Build history of the part. All positions in model axes, mm. A direction names the side the tool comes from. Coordinates: 2 decimals unless noted, no trailing zeros. Loops run counter-clockwise (first coordinate to the right, second up) from the corner with the lowest first, then second, coordinate; pieces in that order, holes last.
(1) Tool access for faces 1 (the face through (3.113, 21, 75)), 2 (the face through (2.98, -5.72, 35.74)), 3 (the face through (21, -3.014, 75)), 4 (the face through (-11.93, -17.92, 75.04)), 5 (the face through (-16.65, 13.33, 75.04)): list every direction of +Z, -Z, +X, -X, +Y, -Y with a clear straight run to the whole face (end or side of a thin tool).
(2) Slice it at B-B (y = 21). Give the cut face in (x, z).
(3) Slice it at C-C (y = 5). Give the cut face in (x, z), and give its area (3 significant figures).
(4) Slice it at D-D (z = 24). Give the cut face in (x, y).
(5) Wall check: L1, parallel to Z at x = 0, y = -29; L2, parallel to X at y = 0.5, z = 34.5; L3, parallel to Y at x = 3.5, z = 53. Give the ranges that are in metal, low to high.
(6) Two-plate mould, pull along Y, no slides. Class faces 6 (the face through (-22, -3.014, 75)), 7 (the face through (-3.113, -21, 75)), 8 (the face through (12.71, 18.56, 75.04)): pulls with the +Y half, pulls with the -Y half, needs draft (parallel to the pull), parting line crosses it, or undercut.
(7) Slice it at A-A (x = 11). Give the cut face in (y, z), and give its area (3 significant figures).
(8) Flat gauge pins, fed straight in: P1, Ø1.5, axis at x = -16.5, z = 74, coming from the -Y side; P2, Ø6, axis at x = 3.5, z = -1.5, coming from the -Y side; P3, Ø1.5, axis at x = 18.5, z = 76, coming from the -Y side; P4, Ø8, axis at x = 11.5, z = 65, coming from the +Y side. Where does each tip first touch, or does it go through?
from build123d import *

# Parameters (mm, degrees)
F0_R     = 6.448973
F1_DEPTH = 75
F3_DEPTH = 2.5
F4_R     = 0.829457
F5_DEPTH = 10
F6_R     = 2.985261
F7_DEPTH = 2


with BuildPart() as f1:
    # F0 (on Top) → F1 (new body)
    with BuildSketch(Plane.XY):
        Circle(F0_R)
    extrude(amount=F1_DEPTH)

    # F2 (on face) → F3 (join, symmetric)
    with BuildSketch(Plane.XY.offset(75)):
        Polygon((7.441463, -3.014468), (35.017251, -3.014468), (35.017251, 3.014468), (8.35262, 3.014468), (27.479934, 22.758793), (22.040198, 28.188686), (3.112997, 8.650931), (3.112997, 33.119855), (-3.112997, 33.119855), (-3.112997, 9.167791), (-19.670232, 28.278624), (-25.342984, 23.363868), (-7.712681, 3.014468), (-35.017251, 3.014468), (-35.017251, -3.014468), (-8.187858, -3.014468), (-26.021978, -21.423882), (-20.502207, -26.77116), (-3.112997, -8.821007), (-3.112997, -33.119855), (3.112997, -33.119855), (3.112997, -9.480839), (20.888046, -29.997309), (26.634359, -25.167458), align=None)
    extrude(amount=F3_DEPTH, both=True)

    # F4 (on face) → F5 (join)
    with BuildSketch(Plane(origin=(0, 0, 0), x_dir=(1, 0, 0), z_dir=(0, 0, -1))):
        Circle(F4_R)
    extrude(amount=F5_DEPTH)

    # F6 (on face) → F7 (join)
    with BuildSketch(Plane(origin=(0, 0, -10), x_dir=(1, 0, 0), z_dir=(0, 0, -1))):
        Circle(F6_R)
    extrude(amount=F7_DEPTH)


solid = f1.part
Response values:
1. face 1: +Z, -Z, +Y
1. face 2: -Z
1. face 3: +Z, -Z, +X
1. face 4: +Z, -Z, -Y
1. face 5: +Z, -Z, -X
2. outline: (-23.29, 72.5) - (-13.36, 72.5) - (-13.36, 77.5) - (-23.29, 77.5) - close; (-3.11, 72.5) - (3.11, 72.5) - (3.11, 77.5) - (-3.11, 77.5) - close; (15.08, 72.5) - (25.78, 72.5) - (25.78, 77.5) - (15.08, 77.5) - close
3. outline: (-9.43, 72.5) - (-4.07, 72.5) - (-4.07, 0) - (4.07, 0) - (4.07, 72.5) - (10.28, 72.5) - (10.28, 77.5) - (-9.43, 77.5) - close
3. area: 689 mm2
4. outline: circle Ø12.9 at (0, 0)
5. L1: z = 72.5 to 77.5
5. L2: x = -6.43 to 6.43
5. L3: y = -5.42 to 5.42
6. face 6: undercut
6. face 7: needs draft
6. face 8: pulls with the +Y half
7. outline: (-18.58, 72.5) - (-7.12, 72.5) - (-7.12, 77.5) - (-18.58, 77.5) - close; (-3.01, 72.5) - (3.01, 72.5) - (3.01, 77.5) - (-3.01, 77.5) - close; (5.75, 72.5) - (16.79, 72.5) - (16.79, 77.5) - (5.75, 77.5) - close
7. area: 143 mm2
8. P1: stops at y = -23.41
8. P2: stops at y = -6.39
8. P3: stops at y = -28.11
8. P4: passes through
